from build123d import *

# Parameters (mm, degrees)
ESQUISSE1_W                     = 10
ESQUISSE1_H                     = 10
BOSS_EXTRU_1_DEPTH              = 252
ESQUISSE2_W                     = 10
ESQUISSE2_H                     = 2
ENL_V_MAT_EXTRU_1_DEPTH         = 11
ESQUISSE5_W                     = 2
ESQUISSE5_H                     = 10
ENL_V_MAT_EXTRU_4_DEPTH         = 11
TROU_TARAUD_M3X0_51_D           = 2.5
TROU_TARAUD_M3X0_51_CSINK_D     = 3.05
TROU_TARAUD_M3X0_51_CSINK_ANGLE = 90


with BuildPart() as part:
    # Esquisse1 → Boss.-Extru.1 (new body)
    with BuildSketch(Plane.XY):
        Rectangle(ESQUISSE1_W, ESQUISSE1_H)
    extrude(amount=BOSS_EXTRU_1_DEPTH)

    # Esquisse2 → Enlèv. mat.-Extru.1 (cut, through all)
    with BuildSketch(Plane.ZY.offset(5)):
        with Locations((5, -4)):
            Rectangle(ESQUISSE2_W, ESQUISSE2_H)
        with Locations((57.4, -4)):
            Rectangle(ESQUISSE2_W, ESQUISSE2_H)
        with Locations((247, -4)):
            Rectangle(ESQUISSE2_W, ESQUISSE2_H)
    extrude(amount=-ENL_V_MAT_EXTRU_1_DEPTH, mode=Mode.SUBTRACT)

    # Esquisse5 → Enlèv. mat.-Extru.4 (cut, through all)
    with BuildSketch(Plane(origin=(0, 5, 0), x_dir=(1, 0, 0), z_dir=(0, 1, 0))):
        with Locations((-4, -194.2)):
            Rectangle(ESQUISSE5_W, ESQUISSE5_H)
        with Locations((-4, -31.2)):
            Rectangle(ESQUISSE5_W, ESQUISSE5_H)
    extrude(amount=-ENL_V_MAT_EXTRU_4_DEPTH, mode=Mode.SUBTRACT)

    # Trou taraudé M3x0.51 (through all)
    with Locations(Plane(origin=(0, 5, 0), x_dir=(1, 0, 0), z_dir=(0, 1, 0))):
        with Locations((0, -20), (0, -232)):
            CounterSinkHole(TROU_TARAUD_M3X0_51_D / 2, TROU_TARAUD_M3X0_51_CSINK_D / 2, counter_sink_angle=TROU_TARAUD_M3X0_51_CSINK_ANGLE)


solid = part.part
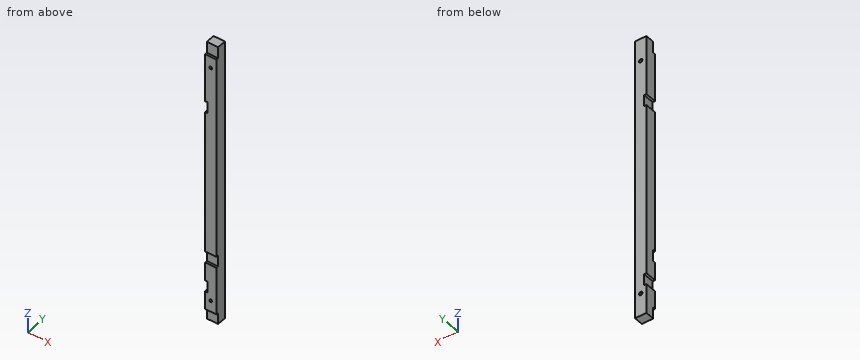
Geometry: final body of the model. Coordinates: model frame, mm. Coordinates: 2 decimals unless noted, no trailing zeros. Order: outer loops, then holes, each group sorted by start corner. A loop starts at its lowest first (then second) coordinate and runs counter-clockwise, first axis right, second up. Notation, with made-up numbers: M -12.75,56 L 17.25,56 A14 ccw 17.25,66 Z; hole C 36.5,78 d8. An arc over 180 degrees is marked long. One line per question, with ' | ' between items. Start each with the question number.
Item 1: Cut plane B-B, the plane z = 54.5. Return the cut outline in (x, y).
Item 2: Pin query (flat end, axial travel): pin 1 Ø0.6 at (x, y) = (0.5, -4.5) entering from -Z; pin 2 Ø2 at (x, y) = (-4.5, -1.5) entering from -Z; pin 3 Ø5 at (x, z) = (0.5, 55) entering from -Y; pin 4 Ø3 at (x, z) = (0, 20) entering from +Y (3 decimals). Return the tip coordinate at first contact, or that it passes through.
Item 3: Ray query, probe 1 along Z at (x, y) = (0, 1.5); probe 2 along Z at (x, y) = (-4.5, 1); probe 3 along X at (y, z) = (-2.5, 20). Return the intervals inside material, ascending. Write a range as [from, to].
Item 4: Cut plane A-A, the plane y = -1. Return the cut outline in (x, z), then the cut area to 3 significant figures.
A:
1) outline: M -5,-3 L 5,-3 L 5,5 L -5,5 Z
2) pin 1: stops at z = 10 | pin 2: stops at z = 0 | pin 3: stops at y = -3 | pin 4: stops at y = 4.975
3) probe 1: z = [0, 18.75], [21.25, 230.75], [233.25, 252] | probe 2: z = [0, 26.2], [36.2, 189.2], [199.2, 252] | probe 3: x = [-5, -1.25], [1.25, 5]
4) outline: M -5,0 L 5,0 L 5,252 L -5,252 L -5,199.2 L -3,199.2 L -3,189.2 L -5,189.2 L -5,36.2 L -3,36.2 L -3,26.2 L -5,26.2 Z; hole C 0,20 d2.5; hole C 0,232 d2.5 | area: 2,470 mm2
